Drawing for the job (mm, zero at the part's lowest x, y, z). Coordinates: 2 decimals unless noted, no trailing zeros. Write each loop counter-clockwise with the first axis right and the second up, starting at its lowest first coordinate (ties: lowest second). Pieces come first, ordered by that corner, then holes. Notation, with made-up numbers: M 35,82.5 L 91,82.5 A35 cw 91,117.5 Z; hole C 80,-3 d9. An arc over 180 degrees is marked long. Use a Markdown table: item, result. Add a question column.
Q1. Slice it at A-A on z = 12.7. Write the cut outline in (x, y) (3 decimals).
Q2. Pin check, flat tips, straight feed: pin 1 Ø3 at (x, y) = (2.5, 11) entering from +Z; pin 2 Ø1.5 at (x, y) = (1, 9.5) entering from -Z; pin 3 Ø1 at (x, y) = (3.5, 20) entering from -Z. Stop position of each tip, or through.
Q3. Slice it at C-C on x = 5. Write the cut outline in (y, z) (3 decimals).
Q4. Slice it at D-D on x = 2.75. Write the cut outline in (y, z) (3 decimals).
Q5. Wall check: L1, parallel to Z at x = 3.25, y = 12.7 (3 decimals); L2, parallel to Z at x = 5.25, y = 11.25; L3, parallel to Y at x = 5, z = 8.25. Give the ranges that are in metal, low to high. Write a range as from..to.
Q6. Mould opens along Y. For the marked faces 1, 2 and 3 say: released by +Y, released by -Y, zero draft, split by the parting line, or undercut.
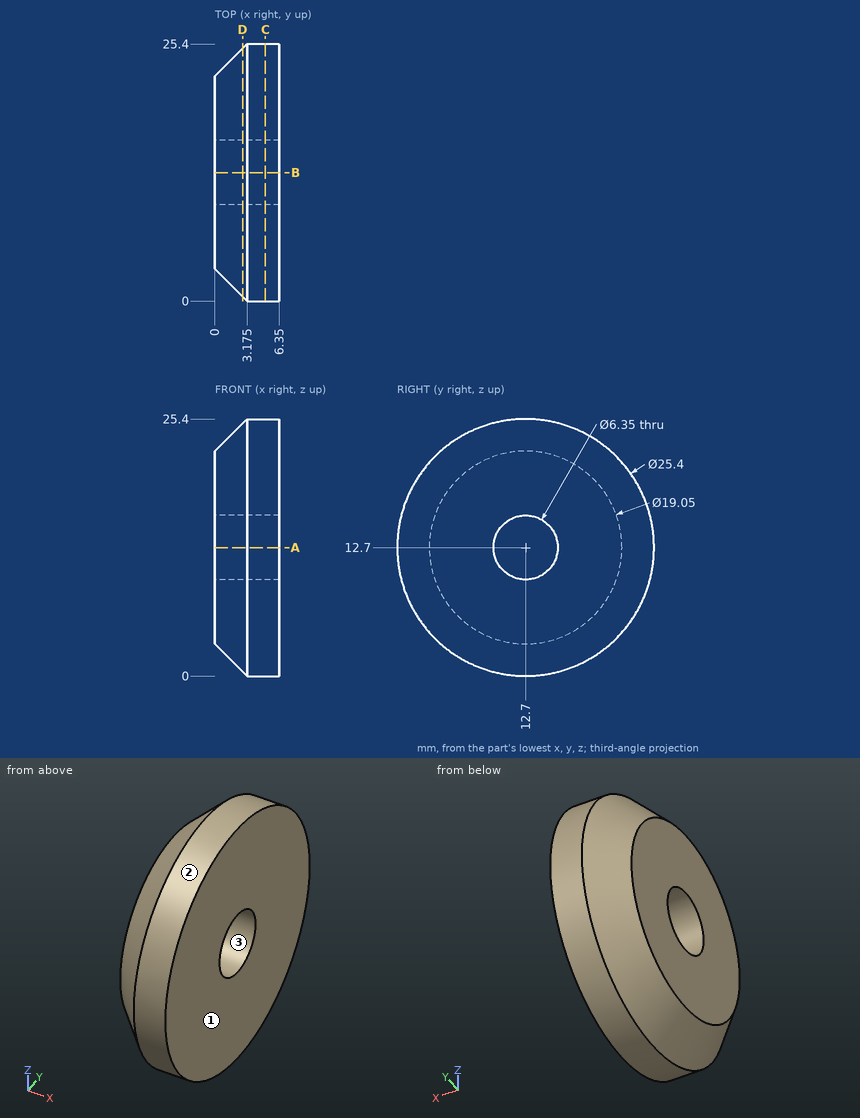
Recorded:
| question | item | result |
|---|---|---|
| 1 | outline | M 0,3.175 L 3.175,0 L 6.35,0 L 6.35,9.525 L 0,9.525 Z; M 0,15.875 L 6.35,15.875 L 6.35,25.4 L 3.175,25.4 L 0,22.225 Z |
| 2 | pin 1 | z = 25.39 |
| 2 | pin 2 | z = 1.86 |
| 2 | pin 3 | z = 1.97 |
| 3 | outline | C 12.7,12.7 d25.4; hole C 12.7,12.7 d6.35 |
| 4 | outline | C 12.7,12.7 d24.55; hole C 12.7,12.7 d6.35 |
| 5 | L1 | 0..9.525, 15.875..25.4 |
| 5 | L2 | 0.08..9.88, 15.52..25.32 |
| 5 | L3 | 0.81..24.59 |
| 6 | face 1 | zero draft |
| 6 | face 2 | split by the parting line |
| 6 | face 3 | undercut |
